```python
from build123d import *

# Parameters (mm, degrees)
SKETCH_1_W           = 260
SKETCH_1_H           = 275
EXTRUDE_1_DEPTH      = 107
EXTRUDE_2_DEPTH      = 25
EXTRUDE_2_DEPTH_BACK = 100
SKETCH_2_R           = 37.5
SKETCH_3_W           = 180.515861549
SKETCH_3_H           = 15
CUT_EXTRUDE_1_DEPTH  = 398.171562426
M4X0_7_1_D           = 3.3
M4X0_7_1_DEPTH       = 11.5
M4X0_7_1_TIP         = 0.991420021
M4X0_7_2_D           = 3.3
M4X0_7_2_DEPTH       = 11.5
M4X0_7_2_TIP         = 0.991420021
SKETCH_17_R          = 37.5
SKETCH_17_R_2        = 33.067386868
EXTRUDE_4_DEPTH      = 20


with BuildPart() as part:
    # 스케치1 → 보스-돌출1 (new body)
    with BuildSketch(Plane(origin=(0, 0, 0), x_dir=(1, 0, 0), z_dir=(0, 1, 0))):
        with Locations((130, 137.5)):
            Rectangle(SKETCH_1_W, SKETCH_1_H)
    extrude(amount=EXTRUDE_1_DEPTH)

    # 스케치2 → 보스-돌출2 (add, two sides: drawn at the far end of the back side and taken through both)
    with BuildSketch(Plane.XY.offset(-EXTRUDE_2_DEPTH_BACK)):
        with Locations((203, 83)):
            Circle(SKETCH_2_R)
    extrude(amount=EXTRUDE_2_DEPTH + EXTRUDE_2_DEPTH_BACK)

    # 스케치3 → 컷-돌출1 (cut, through all)
    with BuildSketch(Plane(origin=(260, 0, 0), x_dir=(0, 0, -1), z_dir=(1, 0, 0))):
        with Locations((184.742069226, 7.5)):
            Rectangle(SKETCH_3_W, SKETCH_3_H)
    extrude(amount=-CUT_EXTRUDE_1_DEPTH, mode=Mode.SUBTRACT)

    # M4x0.7 나사 구멍1
    with Locations(Plane(origin=(0, 15, 0), x_dir=(-1, 0, 0), z_dir=(0, -1, 0))):
        with Locations((-36, 235), (-209, 235)):
            Hole(M4X0_7_1_D / 2, depth=M4X0_7_1_DEPTH)
            with Locations((0, 0, -(M4X0_7_1_DEPTH + M4X0_7_1_TIP / 2))):  # 118° drill point
                Cone(0, M4X0_7_1_D / 2, M4X0_7_1_TIP, mode=Mode.SUBTRACT)

    # M4x0.7 나사 구멍2
    with Locations(Plane(origin=(0, 0, 0), x_dir=(-1, 0, 0), z_dir=(0, -1, 0))):
        with Locations((-142, 47)):
            Hole(M4X0_7_2_D / 2, depth=M4X0_7_2_DEPTH)
            with Locations((0, 0, -(M4X0_7_2_DEPTH + M4X0_7_2_TIP / 2))):  # 118° drill point
                Cone(0, M4X0_7_2_D / 2, M4X0_7_2_TIP, mode=Mode.SUBTRACT)

    # 스케치17 → 보스-돌출4 (add)
    with BuildSketch(Plane.XY.offset(25)):
        with Locations((203, 83)):
            Circle(SKETCH_17_R)
        with Locations((203, 83)):
            Circle(SKETCH_17_R_2, mode=Mode.SUBTRACT)
    extrude(amount=EXTRUDE_4_DEPTH)


solid = part.part
```
Geometry: final body of the model. Coordinates: model frame, mm. A direction names the side the tool comes from. Give positions to 0.01 mm unless a question says otherwise; leave off trailing zeros. Loops run counter-clockwise (first coordinate to the right, second up) from the corner with the lowest first, then second, coordinate; pieces in that order, holes last. Notation, with made-up numbers: (77, -34) -> (94, -34) arc R19 cw to (94, 0) -> close; hole circle Ø1 at (79, -36.5). An arc over 180 degrees is marked (long way). Return JSON: item names as keys, results as strings.
Item 1: Line query: line 1 (X direction, y = 17, z = -235); line 2 (Z direction, x = 36, y = 24); line 3 (X direction, y = 83.5, z = 28). Output: solid intervals per line, ascending.
Filled in:
{"line 1": "0 to 34.35, 37.65 to 207.35, 210.65 to 260", "line 2": "-275 to -236.65, -233.35 to 0", "line 3": "165.5 to 169.94, 236.06 to 240.5"}
Item 2: Mould query, pull axis Y, two halves, no side actions, for faces 1 (the flat face through (0, 53, -136)), 2 (the flat face through (128, 0, -48)), 3 (the cylindrical face through (198.12, 120.18, -12.4)), 4 (the cylindrical face through (176.76, 62.88, 34.86)). Classes: released by +Y, released by -Y, zero draft, split by the parting line, or undercut.
Filled in:
{"face 1": "zero draft", "face 2": "released by -Y", "face 3": "split by the parting line", "face 4": "undercut"}
Item 3: Access query for faces 5 (the flat face through (205.6, 49.8, 45)), 6 (the flat face through (203, 83, 25)), 7 (the flat face through (260, 53, -136)), 8 (the flat face through (132, 7, -94.484)), 9 (the flat face through (203, 112, -100)). Directions: +Z, -Z, +X, -X, +Y, -Y. A direction counts if a zero-diameter tool reaches every point of the face in a straight line with its end or side. Return the directions, or none.
Filled in:
{"face 5": "+Z, +X, -X, +Y, -Y", "face 6": "+Z", "face 7": "+Z, -Z, +X, +Y, -Y", "face 8": "-Z, +X, -X, -Y", "face 9": "-Z, +X, -X, +Y"}
Item 4: Section D-D, the plane y = 31.5. Output: boundary loops of the cut face in (x, z), plus the area to 3 significant figures.
Filled in:
{"outline": "(0, -275) -> (260, -275) -> (260, 0) -> (0, 0) -> close", "area": "71,500 mm^2"}
Item 5: Section A-A, the plane y = 83. Output: boundary loops of the cut face in (x, z), plus the area to 3 significant figures.
Filled in:
{"outline": "(0, -275) -> (260, -275) -> (260, 0) -> (240.5, 0) -> (240.5, 45) -> (236.07, 45) -> (236.07, 25) -> (169.93, 25) -> (169.93, 45) -> (165.5, 45) -> (165.5, 0) -> (0, 0) -> close", "area": "73,600 mm^2"}
Item 6: Pin query (flat end, axial travel): P1, Ø3, axis at x = 209, z = -235, coming from the -Y side; P2, Ø4, axis at x = 54, z = -178, coming from the +Y side; P3, Ø4.5, axis at x = 169.5, y = 7, coming from the -Z side. Return the tip coordinate at first contact, or that it passes through.
Filled in:
{"P1": "y = 26.59", "P2": "y = 107", "P3": "z = -94.48"}
Item 7: Section B-B, the plane x = 107. Output: boundary loops of the cut face in (y, z), plus the area to 3 significant figures.
Filled in:
{"outline": "(0, -94.48) -> (15, -94.48) -> (15, -275) -> (107, -275) -> (107, 0) -> (0, 0) -> close", "area": "26,700 mm^2"}
Item 8: Section C-C, the plane z = -4. Output: boundary loops of the cut face in (x, y).
Filled in:
{"outline": "(0, 0) -> (260, 0) -> (260, 107) -> (231.81, 107) arc R37.5 ccw to (174.19, 107) -> (0, 107) -> close"}
